Could you check a few things on this model? Use its own coordinates, in mm. Coordinates: 2 decimals unless noted, no trailing zeros. Order: outer loops, then holes, each group sorted by start corner. A loop starts at its lowest first (then second) coordinate and runs counter-clockwise, first axis right, second up. Notation, with made-up numbers: (89, 20) - (120, 20) arc R15 ccw to (120, 34) - close; hole circle Ø11 at (6, 36.5). An arc over 180 degrees is marked (long way). Answer as CSV lines item,"result". Start each with the question number.
1. I want a section at D-D, the plane y = 23. List the corners of the cut face in (x, z) for me, and give its area (3 significant figures).
2. I need wall thicknesses on probe 1 along Y at (x, z) = (-3, 2); probe 2 along X at (y, z) = (10, 7.5); probe 3 along Y at (x, z) = (0, 4.25). Which ranges of each line are inside material? Lowest first, please.
3. I want a section at A-A, the plane y = -106.5. List the corners of the cut face in (x, z) for me.
4. I want a section at B-B, the plane x = 3.5. List the corners of the cut face in (y, z) for me, and give its area (3 significant figures).
5. For pin 1 (6 mm diameter, centred on x = 34.5, z = 5, fed in from -Y); pin 2 (3 mm diameter, centred on x = -72.5, z = 4, fed in from -Y); pin 3 (1.5 mm diameter, centred on y = -105.5, z = 2, fed in from +X), each with a flat end and sliding along its axis, tell me the tip position at first contact or that it passes through.
6. I want a section at C-C, the plane z = 7. List the corners of the cut face in (x, y) for me.
from build123d import *

# Parameters (mm, degrees)
ESQUISSE1_R        = 40.5
ESQUISSE1_R_2      = 6
BOSS_EXTRU_1_DEPTH = 10


with BuildPart() as part:
    # Esquisse1 → Boss.-Extru.1 (new body)
    with BuildSketch(Plane.XY):
        with BuildLine():
            Line((-25, -140), (-10, -140))
            Line((-10, -140), (60.378177886, -44.49129842))
            ThreePointArc((60.378177886, -44.49129842), (47.149121788, 58.326326085), (-56.15757152, 49.712444729))
            Line((-56.15757152, 49.712444729), (-140, -45))
            Line((-140, -45), (-140, -140))
            Line((-140, -140), (-125, -140))
            Line((-125, -140), (-125, -60))
            Line((-125, -60), (-25, -60))
            Line((-25, -60), (-25, -140))
        make_face()
        Circle(ESQUISSE1_R, mode=Mode.SUBTRACT)
        with Locations((-49.686682345, 5.520742483)):
            Circle(ESQUISSE1_R_2, mode=Mode.SUBTRACT)
        with Locations((5.520742483, 49.686682345)):
            Circle(ESQUISSE1_R_2, mode=Mode.SUBTRACT)
        with Locations((49.686682345, -5.520742483)):
            Circle(ESQUISSE1_R_2, mode=Mode.SUBTRACT)
        with Locations((-5.520742483, -49.686682345)):
            Circle(ESQUISSE1_R_2, mode=Mode.SUBTRACT)
    extrude(amount=BOSS_EXTRU_1_DEPTH)


solid = part.part
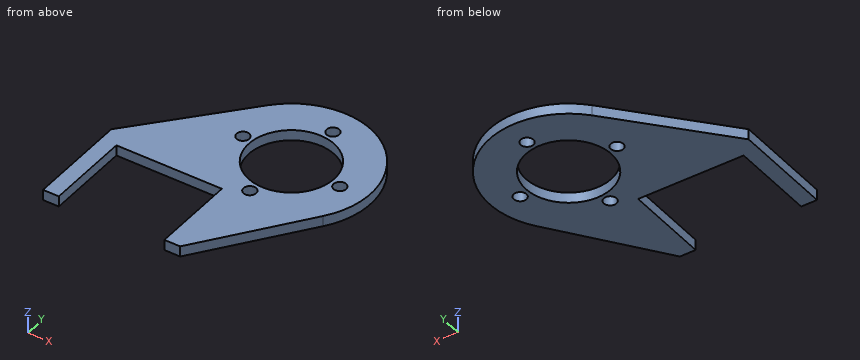
Solved:
1,outline,"(-79.8, 0) - (-33.34, 0) - (-33.34, 10) - (-79.8, 10) - close; (33.34, 0) - (71.39, 0) - (71.39, 10) - (33.34, 10) - close"
1,area,"845 mm2"
2,probe 1,"y = -130.5 to -55.13, -44.24 to -40.39, 40.39 to 74.94"
2,probe 2,"x = -91.31 to -53.68, -45.69 to -39.25, 39.25 to 74.33"
2,probe 3,"y = -126.43 to -52.04, -47.34 to -40.5, 40.5 to 47.34, 52.04 to 75"
3,outline,"(-140, 0) - (-125, 0) - (-125, 10) - (-140, 10) - close; (-25, 0) - (14.69, 0) - (14.69, 10) - (-25, 10) - close"
4,outline,"(-121.68, 0) - (-40.35, 0) - (-40.35, 10) - (-121.68, 10) - close; (40.35, 0) - (44.04, 0) - (44.04, 10) - (40.35, 10) - close; (55.34, 0) - (74.92, 0) - (74.92, 10) - (55.34, 10) - close"
4,area,"1,050 mm2"
5,pin 1,"stops at y = -83.68"
5,pin 2,"stops at y = -60"
5,pin 3,"stops at x = 15.97"
6,outline,"(-140, -140) - (-125, -140) - (-125, -60) - (-25, -60) - (-25, -140) - (-10, -140) - (60.38, -44.49) arc R75 ccw to (-56.16, 49.71) - (-140, -45) - close; hole circle Ø12 at (-49.69, 5.52); hole circle Ø81 at (0, 0); hole circle Ø12 at (-5.52, -49.69); hole circle Ø12 at (5.52, 49.69); hole circle Ø12 at (49.69, -5.52)"
